Can you work these out from the model? Positions are in its coordinate system, mm. A direction names the side the tool comes from. Coordinates: 2 decimals unless noted, no trailing zeros. Order: outer loops, then holes, each group sorted by start corner. A loop starts at its lowest first (then second) coordinate and runs counter-clockwise, first axis right, second up. Notation, with made-up numbers: (-19, 15.25) -> (-8, 15.25) arc R19 cw to (-8, 34.25) -> close; hole circle Ø7 at (-30.75, 1.5). An arc over 180 degrees is marked (long way). Use a Markdown table: item, result. Add a question column.
1. Suppose I cut it at C-C, the plane z = 39. List the corners of the cut face in (x, y) for me.
2. If I drill on line 1 along Z through (x, y) = (-16.5, 23.5); line 2 along X through (y, z) = (1, 46); line 3 along X through (y, z) = (11, 184), over which ranges is the centre line in solid material (lowest first)? Write a range as from..to.
3. For pin 1 Ø3 at (x, z) = (1, 247) entering from +Y; pin 2 Ø8 at (y, z) = (-10.5, 436) entering from -X; pin 3 Ø8 at (x, y) = (-21.5, 20.5) entering from -Z; pin 4 Ø5 at (y, z) = (-18, 313.5) entering from -X, each with a flat end and sliding along its axis, tell me the tip position at first contact or that it passes through.
4. Suppose I cut it at A-A, the plane y = 0. List the corners of the cut face in (x, z) for me.
5. Suppose I cut it at D-D, the plane y = 22.5. List the corners of the cut face in (x, z) for me.
6. For faces 1 (the flat face through (0, 0, 503)), 2 (the flat face through (-7, 14, 500)), which set-ups out of +Z, -Z, +X, -X, +Y, -Y let a thin tool reach every point of the face, with its end or its side?
```python
from build123d import *

# Parameters (mm, degrees)
F0_R     = 15
F1_DEPTH = 500
F2_W     = 60
F2_H     = 60
F2_R     = 15
F3_DEPTH = 3


with BuildPart() as f1:
    # F0 (on Top) → F1 (new body)
    with BuildSketch(Plane.XY):
        Circle(F0_R)
    extrude(amount=F1_DEPTH)

    # F2 (on face) → F3 (join)
    with BuildSketch(Plane.XY.offset(500)):
        Rectangle(F2_W, F2_H)
        Circle(F2_R, mode=Mode.SUBTRACT)
        Rectangle(F2_W, F2_H)
    extrude(amount=F3_DEPTH)


solid = f1.part
```
Worked out:
| question | item | result |
|---|---|---|
| 1 | outline | circle Ø30 at (0, 0) |
| 2 | line 1 | z = 500..503 |
| 2 | line 2 | x = -14.97..14.97 |
| 2 | line 3 | x = -10.2..10.2 |
| 3 | pin 1 | stops at y = 15 |
| 3 | pin 2 | stops at x = -13.52 |
| 3 | pin 3 | stops at z = 500 |
| 3 | pin 4 | passes through |
| 4 | outline | (-30, 500) -> (-15, 500) -> (-15, 0) -> (15, 0) -> (15, 500) -> (30, 500) -> (30, 503) -> (-30, 503) -> close |
| 5 | outline | (-30, 500) -> (30, 500) -> (30, 503) -> (-30, 503) -> close |
| 6 | face 1 | +Z, +X, -X, +Y, -Y |
| 6 | face 2 | -Z |
